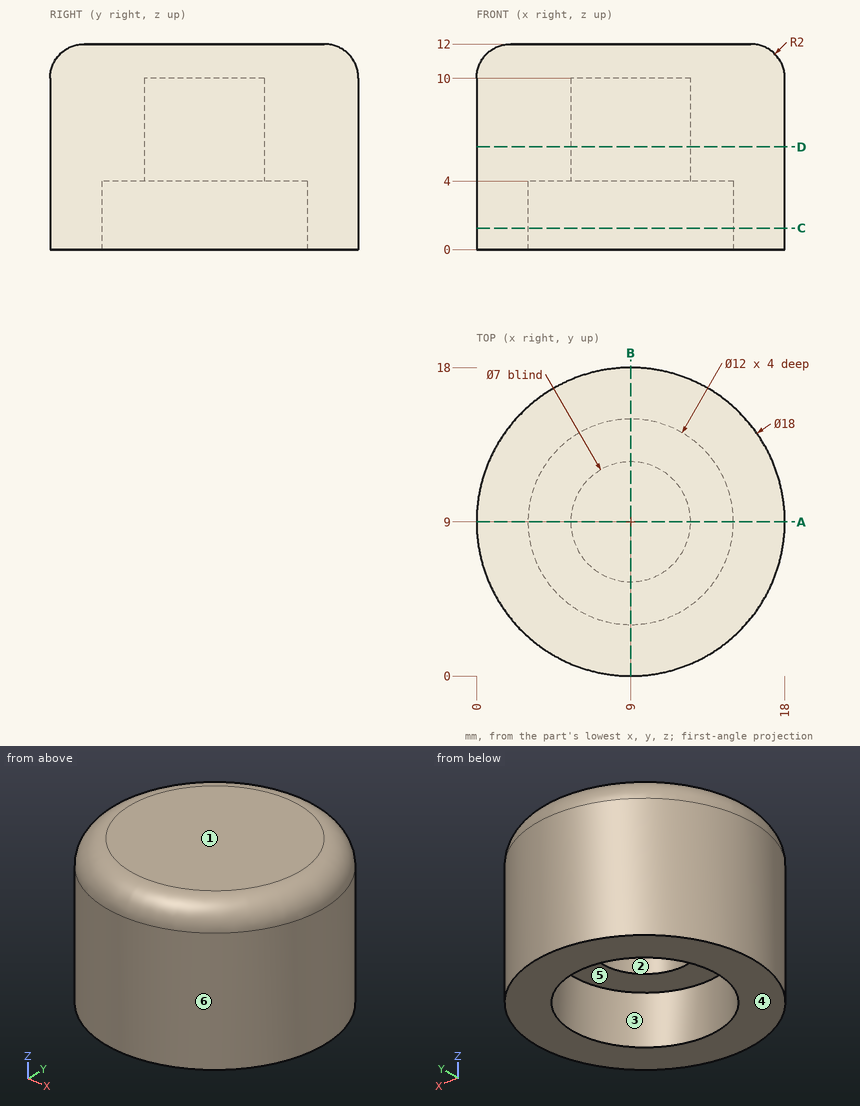
Can you work these out from the drawing? Everything is in mm from the part's minimum corner. A direction names the side the tool comes from. Give positions to 0.01 mm unless a question says otherwise; leave off trailing zeros. Write each loop counter-clockwise with the first axis right and the second up, starting at its lowest first coordinate (ties: lowest second). Pieces come first, ordered by that corner, then holes. Notation, with made-up numbers: (51.5, 64) -> (89.5, 64) arc R18 cw to (89.5, 69) -> close; hole circle Ø8 at (34, 73). An arc over 180 degrees is marked (long way). Write each question's results on one line, items separated by ' | '. Start each with the question number.
Q1. Suppose I cut it at C-C, the plane z = 1.25. List the corners of the cut face in (x, y) for me.
Q2. I need wall thicknesses on probe 1 along Y at (x, z) = (9, 8.55); probe 2 along Y at (x, z) = (9, 2.65); probe 3 along Z at (x, y) = (4.75, 6.25). Which ranges of each line are inside material? Lowest first, please.
Q3. Which directions (+Z, -Z, +X, -X, +Y, -Y) give clear straight access to the entire face, cutting with the end or side of a thin tool? Please do the marked faces 1 and 2.
Q4. Suppose I cut it at D-D, the plane z = 6. List the corners of the cut face in (x, y) for me.
Q5. We'd pull the mould along X, two halves only. Please class the marked faces 3, 4, 5 and 6: +X half, -X half, draft (parallel to the pull), parting line (faces both ways), or undercut.
Q6. I'm going to push flat-ended pins straight in: pin 1 Ø7.5 at (x, y) = (8, 8.5) entering from -Z; pin 2 Ø2 at (x, y) = (3, 14.5) entering from -Z; pin 3 Ø3 at (x, z) = (4.5, 8.5) entering from +Y; pin 4 Ø1 at (y, z) = (12.5, 6.5) entering from +X. Where does each tip first touch, or does it pass through?
Q7. Suppose I cut it at A-A, the plane y = 9. List the corners of the cut face in (x, z) for me, and give its area (3 significant figures).
Outcome:
1) outline: circle Ø18 at (9, 9); hole circle Ø12 at (9, 9)
2) probe 1: 0 to 5.5, 12.5 to 18 | probe 2: 0 to 3, 15 to 18 | probe 3: 4 to 12
3) face 1: +Z, +X, -X, +Y, -Y | face 2: -Z
4) outline: circle Ø18 at (9, 9); hole circle Ø7 at (9, 9)
5) face 3: undercut | face 4: draft | face 5: undercut | face 6: parting line
6) pin 1: z = 4 | pin 2: z = 0 | pin 3: y = 17.49 | pin 4: x = 17.49
7) outline: (0, 0) -> (3, 0) -> (3, 4) -> (5.5, 4) -> (5.5, 10) -> (12.5, 10) -> (12.5, 4) -> (15, 4) -> (15, 0) -> (18, 0) -> (18, 10) arc R2 ccw to (16, 12) -> (2, 12) arc R2 ccw to (0, 10) -> close | area: 124 mm2
